from build123d import *

# Parameters (mm, degrees)
F0_W     = 31.75
F0_H     = 31.75
F1_DEPTH = 44.45
F2_W     = 12.7
F2_H     = 12.7
F3_DEPTH = 63.5
F4_W     = 31.75
F4_H     = 12.7
F5_DEPTH = 6.35
F6_W     = 12.7
F6_H     = 12.7
F6_W_2   = 6.35
F7_DEPTH = 31.75


with BuildPart() as f1:
    # F0 (on Top) → F1 (new body, symmetric)
    with BuildSketch(Plane.XY):
        Rectangle(F0_W, F0_H)
    extrude(amount=F1_DEPTH, both=True)

    # F2 (on face) → F3 (join)
    with BuildSketch(Plane(origin=(0, 0, -44.45), x_dir=(1, 0, 0), z_dir=(0, 0, -1))):
        Rectangle(F2_W, F2_H)
    extrude(amount=F3_DEPTH)

    # F4 (on face) → F5 (cut)
    with BuildSketch(Plane.XY.offset(44.45)):
        Rectangle(F4_W, F4_H)
    extrude(amount=-F5_DEPTH, mode=Mode.SUBTRACT)

    # F6 (on face) → F7 (cut, through all)
    with BuildSketch(Plane.YZ.offset(15.875)):
        with Locations((9.525, 19.05)):
            Rectangle(F6_W, F6_H)
        with Locations((12.7, -25.4)):
            Rectangle(F6_W_2, F6_H)
        with Locations((-9.525, -25.4)):
            Rectangle(F6_W, F6_H)
        with Locations((-12.7, 19.05)):
            Rectangle(F6_W_2, F6_H)
    extrude(amount=-F7_DEPTH, mode=Mode.SUBTRACT)


solid = f1.part
Check sheet for the modelled part. Datum: model origin and axes. Units: mm. A direction names the side the tool comes from. Give positions to 0.01 mm unless a question says otherwise; leave off trailing zeros. Loops run counter-clockwise (first coordinate to the right, second up) from the corner with the lowest first, then second, coordinate; pieces in that order, holes last. Notation, with made-up numbers: M 50.5,51.25 L 99.5,51.25 A12 cw 99.5,62.25 Z; hole C -5.5,56.5 d9. An arc over 180 degrees is marked long. Answer as a JSON object with one key per item and string values. Group by question number.
Q1. Access from +Z, -Z, +X, -X, +Y, -Y to the whole of each face (thin tool, end or side, straight path). Record for faces 1 (the flat face through (0, 9, 25.4)), 2 (the flat face through (0, 6.35, 41)), 3 (the flat face through (-6.35, 0, -76)), 4 (the flat face through (0, -13, 25.4)).
Q2. Cross-section at A-A on y = 8. Record the cut outline in (x, z) (3 decimals).
Q3. Release check for a two-part mould opening along Y. For faces 5 (the flat face through (0, -10, -19.05)), 6 (the flat face through (0, -9.525, 19)), 7 (the flat face through (0, 0, 38.1)) record: released by +Y, released by -Y, zero draft, split by the parting line, or undercut.
Q4. Cross-section at C-C on y = -1.5. Record the cut outline in (x, z) (3 decimals).
Q5. Go/stop test with flat-tipped pins: P1, Ø10, axis at x = 3, z = -84, coming from the +Y side; P2, Ø2, axis at x = -12, z = -25.5, coming from the -Y side (3 decimals); P3, Ø14, axis at y = -0.5, z = -92, coming from the -X side. Record where each tip stops, or that it passes through.
Q6. Cross-section at D-D on z = -22. Record the cut outline in (x, y) (3 decimals), then the cut area to 3 significant figures.
Q7. Material ranges on line 1 along Z through (x, y) = (-2.5, -11); line 2 along Z through (x, y) = (-14, 7); line 3 along X through (y, z) = (-5.5, -60.5), recorded low to high. Write a range as [from, to].
Q8. Cross-section at B-B on x = -10. Record the cut outline in (y, z) (3 decimals), then the cut area to 3 significant figures.
Evaluation:
{
 "1": {"face 1": "+X, -X, +Y", "face 2": "+Z, +X, -X", "face 3": "-Z, -X, +Y, -Y", "face 4": "+X, -X, -Y"},
 "2": {"outline": "M -15.875,-44.45 L 15.875,-44.45 L 15.875,12.7 L -15.875,12.7 Z; M -15.875,25.4 L 15.875,25.4 L 15.875,44.45 L -15.875,44.45 Z"},
 "3": {"face 5": "zero draft", "face 6": "released by -Y", "face 7": "undercut"},
 "4": {"outline": "M -15.875,-44.45 L -6.35,-44.45 L -6.35,-107.95 L 6.35,-107.95 L 6.35,-44.45 L 15.875,-44.45 L 15.875,38.1 L -15.875,38.1 Z"},
 "5": {"P1": "stops at y = 6.35", "P2": "stops at y = -3.175", "P3": "stops at x = -6.35"},
 "6": {"outline": "M -15.875,-3.175 L 15.875,-3.175 L 15.875,9.525 L -15.875,9.525 Z", "area": "403 mm2"},
 "7": {"line 1": "z = [-44.45, -31.75], [-19.05, 12.7], [25.4, 44.45]", "line 2": "z = [-44.45, 12.7], [25.4, 44.45]", "line 3": "x = [-6.35, 6.35]"},
 "8": {"outline": "M -15.875,-44.45 L 15.875,-44.45 L 15.875,-31.75 L 9.525,-31.75 L 9.525,-19.05 L 15.875,-19.05 L 15.875,12.7 L 3.175,12.7 L 3.175,25.4 L 15.875,25.4 L 15.875,44.45 L 6.35,44.45 L 6.35,38.1 L -6.35,38.1 L -6.35,44.45 L -15.875,44.45 L -15.875,25.4 L -9.525,25.4 L -9.525,12.7 L -15.875,12.7 L -15.875,-19.05 L -3.175,-19.05 L -3.175,-31.75 L -15.875,-31.75 Z", "area": "2,260 mm2"}
}
